from build123d import *

# Parameters (mm, degrees)
F1_DEPTH = 63.5
F0_W     = 25.4
F0_H     = 19.05
F2_DEPTH = 25.4
F3_DEPTH = 7.9375
F5_R     = 8.89


with BuildPart() as f1:
    # F0 (on Front) → F1 (new body, symmetric)
    with BuildSketch(Plane.XZ):
        Polygon((-41.275, 9.525), (-41.275, -9.525), (41.275, -9.525), (41.275, 9.525), (22.225, 9.525), align=None)
    extrude(amount=F1_DEPTH, both=True)

    # F0 (on Front) → F2 (join, symmetric)
    with BuildSketch(Plane.XZ):
        with Locations((73.025, 52.4002)):
            Rectangle(F0_W, F0_H)
        with BuildLine():
            Line((22.225, 9.525), (41.275, 9.525))
            Line((41.275, 9.525), (41.275, 27.0005395917))
            ThreePointArc((41.275, 27.0005395917), (45.8880281066, 38.1890879368), (57.0461639775, 42.8752))
            Line((57.0461639775, 42.8752), (60.325, 42.8752))
            Line((60.325, 42.8752), (60.325, 61.9252))
            Line((60.325, 61.9252), (56.9959858401, 61.9252))
            add(Edge.make_bspline(
                [(55.4406243802, 61.8836825118), (55.9614433342, 61.9018413626), (56.4799445563, 61.9157023789), (56.9959858401, 61.9252)],
                knots=[109.9747025798, 109.9747025798, 109.9747025798, 109.9747025798, 111.3686114577, 111.3686114577, 111.3686114577, 111.3686114577], degree=3))
            ThreePointArc((55.4406243802, 61.8836825118), (31.8571594268, 51.0843067542), (22.225, 27.0005395917))
            Line((22.225, 27.0005395917), (22.225, 9.525))
        make_face()
    extrude(amount=F2_DEPTH, both=True)

    # F0 (on Front) → F3 (join, symmetric)
    with BuildSketch(Plane.XZ):
        with BuildLine():
            add(Edge.make_bspline(
                [(-41.275, 9.525), (-41.168221459, 32.2657067872), (14.3497679594, 60.4510105174), (55.4406243802, 61.8836825118)],
                knots=[0, 0, 0, 0, 109.9747025798, 109.9747025798, 109.9747025798, 109.9747025798], degree=3))
            Line((-41.275, 9.525), (22.225, 9.525))
            Line((22.225, 9.525), (22.225, 27.0005395917))
            ThreePointArc((22.225, 27.0005395917), (31.8571594268, 51.0843067542), (55.4406243802, 61.8836825118))
        make_face()
    extrude(amount=F3_DEPTH, both=True)

    # F0 (on Front) → F4 (revolve)
    with BuildSketch(Plane.XZ):
        Polygon((85.725, 66.675), (85.725, 61.9252), (85.725, 42.8752), (85.725, 38.1), (111.125, 38.1), (111.125, 66.675), align=None)
    revolve(axis=Axis((85.725, 0, 52.3875), (0, 0, 1)))

    # F5
    f5_edges = [f1.edges().sort_by_distance(p)[0] for p in [
        (-41.275, -63.5, 0),
        (41.275, -63.5, 0),
        (41.275, 63.5, 0),
        (-41.275, 63.5, 0),
    ]]
    fillet(f5_edges, radius=F5_R)


solid = f1.part
Geometry check sheet. Reference: the model listing, model coordinates, mm. A direction names the side the tool comes from. Give positions to 0.01 mm unless a question says otherwise; leave off trailing zeros. Loops run counter-clockwise (first coordinate to the right, second up) from the corner with the lowest first, then second, coordinate; pieces in that order, holes last.
(1) Depth check by flat-ended pin: pin 1 Ø19 at (y, z) = (-16.5, 19.5) entering from -X; pin 2 Ø6 at (x, z) = (86.5, 44.5) entering from -Y; pin 3 Ø4 at (x, y) = (2, -41.5) entering from +Z (3 decimals). Enter the tip coordinate at first touch or a pass-through.
From the geometry:
pin 1: stops at x = -40.1
pin 2: stops at y = -25.4
pin 3: stops at z = 9.525
(2) Section check A-A on y = 43. Record the cut outline in (x, z) (3 decimals), then the cut area to 3 significant figures.
From the geometry:
outline: (-41.275, -9.525) - (41.275, -9.525) - (41.275, 9.525) - (-41.275, 9.525) - close
area: 1,570 mm2
(3) Set-up check for faces 1 (the cylindrical face through (32.115, -16.791, 51.352)), 2 (the cylindrical face through (45.8, -0.4, 38.1)), 3 (the flat face through (-3, 7.938, 30)), 4 (the flat face through (60, 0, 61.925)), 5 (the flat face through (41.275, -1, 4)): record each of +Z, -Z, +X, -X, +Y, -Y from which the full face is reachable in a straight line by a thin tool's end or side.
From the geometry:
face 1: +Z, -X, -Y
face 2: -Z, +Y, -Y
face 3: +Z, -X, +Y
face 4: +Z, -X
face 5: -Z, +X, +Y, -Y
(4) Thickness scan on L1, parallel to Z at x = 68, y = 25; L2, parallel to X at y = 17, z = 14 (3 decimals); L3, parallel to Z at x = 104.5, y = 16.5 (3 decimals). Record the ranges inside material, lowest first.
From the geometry:
L1: z = 42.88 to 61.93
L2: x = 22.225 to 41.275
L3: z = 38.1 to 66.675
